```python
from build123d import *

# Parameters (mm, degrees)
F0_R           = 30.1625
F1_DEPTH       = 4.318
F2_R           = 34.2265
F2_R_2         = 30.1625
F3_DEPTH       = 17.78
F0_W           = 76.2
F0_H           = 76.2
F0_W_2         = 6.35
F0_H_2         = 6.35
F4_DEPTH       = 2.54
F5_DEPTH       = 11.684
F6_D           = 2.54
F8_D           = 3.175
F8_CSINK_D     = 6.858
F8_CSINK_ANGLE = 90
F9_SIZE        = 2.54
F10_R          = 0.508
F11_R          = 30.1625
F11_R_2        = 29.7565
F12_DEPTH      = 11.6
F13_D          = 5


with BuildPart() as f1:
    # F0 (on Front) → F1 (new body)
    with BuildSketch(Plane.XZ):
        Circle(F0_R)
    extrude(amount=F1_DEPTH)

    # F2 (on Front) → F3 (join)
    with BuildSketch(Plane.XZ):
        Circle(F2_R)
        Circle(F2_R_2, mode=Mode.SUBTRACT)
    extrude(amount=F3_DEPTH)

    # F0 (on Front) → F4 (join)
    with BuildSketch(Plane.XZ):
        Rectangle(F0_W, F0_H)
        with Locations((-31.5595, -31.5595)):
            Rectangle(F0_W_2, F0_H_2, mode=Mode.SUBTRACT)
        with Locations((31.5595, -31.8507122787)):
            Rectangle(F0_W_2, F0_H_2, mode=Mode.SUBTRACT)
        with Locations((-31.5595, 31.5595)):
            Rectangle(F0_W_2, F0_H_2, mode=Mode.SUBTRACT)
        Circle(F0_R, mode=Mode.SUBTRACT)
        with Locations((31.5595, 31.5595)):
            Rectangle(F0_W_2, F0_H_2, mode=Mode.SUBTRACT)
    extrude(amount=F4_DEPTH)

    # F0 (on Front) → F5 (join)
    with BuildSketch(Plane.XZ):
        with Locations((-31.5595, -31.5595)):
            Rectangle(F0_W_2, F0_H_2)
        with Locations((-31.5595, 31.5595)):
            Rectangle(F0_W_2, F0_H_2)
        with Locations((31.5595, 31.5595)):
            Rectangle(F0_W_2, F0_H_2)
        with Locations((31.5595, -31.8507122787)):
            Rectangle(F0_W_2, F0_H_2)
    extrude(amount=F5_DEPTH)

    # F6 (through all)
    with Locations(Plane(origin=(0, 0, 0), x_dir=(1, 0, 0), z_dir=(0, 1, 0))):
        with Locations((-31.5595, -31.5595), (31.5595, -31.5595), (-31.5595, 31.5595), (31.5595, 31.8507122787)):
            Hole(F6_D / 2)

    # F8 (through all)
    with Locations(Plane.XZ.offset(4.318)):
        with Locations((-13.5, -14.1), (13.5, -14.1)):
            CounterSinkHole(F8_D / 2, F8_CSINK_D / 2, counter_sink_angle=F8_CSINK_ANGLE)

    # F9
    f9_edges = [f1.edges().sort_by_distance(p)[0] for p in [
        (-30.1625, -17.78, 0),
    ]]
    chamfer(f9_edges, length=F9_SIZE)

    # F10
    f10_edges = [f1.edges().sort_by_distance(p)[0] for p in [
        (-34.2265, -17.78, 0),
    ]]
    fillet(f10_edges, radius=F10_R)

    # F11 (on Front) → F12 (join)
    with BuildSketch(Plane.XZ):
        Circle(F11_R)
        Circle(F11_R_2, mode=Mode.SUBTRACT)
    extrude(amount=F12_DEPTH)

    # F13 (through all)
    with Locations(Plane.XZ.offset(4.318)):
        with Locations((0, -20.1)):
            Hole(F13_D / 2)


solid = f1.part
```
Geometry check sheet. Reference: the model listing, model coordinates, mm. A direction names the side the tool comes from. Coordinates: 2 decimals unless noted, no trailing zeros. Order: outer loops, then holes, each group sorted by start corner. A loop starts at its lowest first (then second) coordinate and runs counter-clockwise, first axis right, second up. Notation, with made-up numbers: (-39, -31) - (0, -31) arc R9 ccw to (0, -27) - close; hole circle Ø10 at (71, 34.5). An arc over 180 degrees is marked (long way). Answer as a JSON object with one key per item and string values. Group by question number.
Item 1: Draft check along X on faces 6 (the face through (34.734, -7, -32)), 7 (the face through (32, -11.684, 33)), 8 (the face through (-38.1, -1, -1)), 9 (the face through (-30.133, -13.395, 1.326)). Enter one of: +X half, -X half, draft (parallel to the pull), parting line (faces both ways), or undercut.
Item 2: Depth check by flat-ended pin: pin 1 Ø3.5 at (x, z) = (-31.56, 31.56) entering from -Y; pin 2 Ø3 at (x, y) = (-28, -6.5) entering from -Z; pin 3 Ø5 at (y, z) = (-8, 22.5) entering from +X. Enter the tip coordinate at first touch or a pass-through.
Item 3: Tool access check on faces 1 (the face through (32, -7, -35.026)), 2 (the face through (32, -7, 34.734)), 3 (the face through (-30, -11.684, 32)), 4 (the face through (32, -7, 28.384)), 5 (the face through (28.384, -7, 32)). Record the directions out of +Z, -Z, +X, -X, +Y, -Y that give a thin tool (end or side, any length) a straight path to the whole face; none if there is none.
Item 4: Sectioned sample at A-A, the plane x = 0. Record the cut outline in (y, z).
Item 5: Sectioned sample at B-B, the plane z = 0. Record the cut outline in (x, y).
Item 6: Scan lines: probe 1 along Z at (x, y) = (0, -1.9); probe 2 along Z at (x, y) = (0, -9); probe 3 along Z at (x, y) = (-32, -2). Record each from-to range of solid material in increasing order.
Item 7: Sectioned sample at C-C, the plane z = -14.1. Give the number of separate pieces and of enclosed holes in the cut face, and give its area (3 significant figures).
Resolved:
{
 "1": {"face 6": "+X half", "face 7": "draft", "face 8": "-X half", "face 9": "undercut"},
 "2": {"pin 1": "y = -11.68", "pin 2": "z = -34.73", "pin 3": "x = 27.78"},
 "3": {"face 1": "-Z, +X, -X, -Y", "face 2": "+Z, +X, -X, -Y", "face 3": "+Z, -X, -Y", "face 4": "+X, -Y", "face 5": "+Z, -Y"},
 "4": {"outline": "(-17.78, -33.72) arc R0.51 ccw to (-17.27, -34.23) - (-2.54, -34.23) - (-2.54, -38.1) - (0, -38.1) - (0, -22.6) - (-4.32, -22.6) - (-4.32, -29.76) - (-11.6, -29.76) - (-11.6, -30.16) - (-15.24, -30.16) - (-17.78, -32.7) - close; (-17.78, 32.7) - (-15.24, 30.16) - (-11.6, 30.16) - (-11.6, 29.76) - (-4.32, 29.76) - (-4.32, -17.6) - (0, -17.6) - (0, 38.1) - (-2.54, 38.1) - (-2.54, 34.23) - (-17.27, 34.23) arc R0.51 ccw to (-17.78, 33.72) - close"},
 "5": {"outline": "(-38.1, -2.54) - (-34.23, -2.54) - (-34.23, -17.27) arc R0.51 ccw to (-33.72, -17.78) - (-32.7, -17.78) - (-30.16, -15.24) - (-30.16, -11.6) - (-29.76, -11.6) - (-29.76, -4.32) - (29.76, -4.32) - (29.76, -11.6) - (30.16, -11.6) - (30.16, -15.24) - (32.7, -17.78) - (33.72, -17.78) arc R0.51 ccw to (34.23, -17.27) - (34.23, -2.54) - (38.1, -2.54) - (38.1, 0) - (-38.1, 0) - close"},
 "6": {"probe 1": "-38.1 to -22.6, -17.6 to 38.1", "probe 2": "-34.23 to -29.76, 29.76 to 34.23", "probe 3": "-38.1 to -32.75, -30.37 to 30.37, 32.75 to 38.1"},
 "7": {"separate pieces": "3", "enclosed holes": "0", "area": "391 mm^2"}
}
